Source: CAD feature listing. Evaluate the final solid. Frame: model axes, mm. Face numbers are marked on the shaded views. A direction names the side the tool comes from. Give positions to 0.01 mm unless a question says otherwise; leave off trailing zeros. Order: outer loops, then holes, each group sorted by start corner. A loop starts at its lowest first (then second) coordinate and runs counter-clockwise, first axis right, second up. Notation, with made-up numbers: M -0.75,23.25 L 41.25,23.25 A20 ccw 41.25,49.25 Z; hole C 32,-4 d9. An arc over 180 degrees is marked long. Use CSV: the item, a comma, the result in double quotes. Start each with the question number.
Item 1: Pull-direction query (X, two-part tool) for the marked faces 1, 2 and 3; classes: +X half, -X half, draft (parallel to the pull), parting line (faces both ways), or undercut.
Item 2: Section query A-A on y = 25.4. Return loops of the section in (x, z) (3 decimals).
Item 3: Section query C-C on x = 34. Return loops of the section in (y, z).
Item 4: First-contact query: pin 1 (8 mm diameter, centred on x = -3.5, y = 5, fed in from +Z); pin 2 (8 mm diameter, centred on x = -17, z = 72, fed in from +Y); pin 3 (1 mm diameter, centred on x = -32.5, y = 11, fed in from -Z); pin 4 (4 mm diameter, centred on x = 12.5, y = 14.5, fed in from +Z). Flat tips, straight axial feed; report the tip coordinate or a pass-through.
Item 5: Section query D-D on z = 47.5. Return loops of the section in (x, y).
Item 6: Section query B-B on x = 50.8. Return loops of the section in (y, z) (3 decimals), and give its area (3 significant figures).
Item 7: Access query for the marked faces 4 and 5. Directions: +Z, -Z, +X, -X, +Y, -Y. A direction counts if a zero-diameter tool reaches every point of the face in a straight line with its end or side. Return the directions, or none.
Item 8: Ray query, probe 1 along X at (y, z) = (25, 8); probe 2 along Y at (x, z) = (50.8, 8) (3 decimals); probe 3 along X at (y, z) = (-20.5, 4). Return the intervals inside material, ascending. Write a range as from..to.
from build123d import *

# Parameters (mm, degrees)
F0_W     = 127
F0_H     = 76.2
F1_DEPTH = 25.4
F3_D     = 19.05
F4_W     = 19.05
F4_H     = 50.8
F6_W     = 12.7
F6_H     = 25.4
F9_R     = 2.54


# Not quite as in the source:
# - a fillet or chamfer that OpenCascade refuses, or shapes differently, is made with other operations: its cross-section is extruded or revolved along the edge and cut away or added


with BuildPart() as f1:
    # F0 (on Top) → F1 (new body)
    with BuildSketch(Plane.XY):
        Rectangle(F0_W, F0_H)
    extrude(amount=F1_DEPTH)

    # F3 (through all)
    with Locations(Plane.XY.offset(25.4)):
        with Locations((-50.8, 25.4), (50.8, 25.4), (-50.8, -25.4), (50.8, -25.4)):
            Hole(F3_D / 2)

    # F4 (on Front) → F5 (revolve)
    with BuildSketch(Plane.XZ):
        with Locations((-9.525, 50.8)):
            Rectangle(F4_W, F4_H)
    revolve(axis=Axis((0, 0, 50.8), (0, 0, 1)))

    # F6 (on Front) → F7 (revolve, cut)
    with BuildSketch(Plane.XZ):
        with Locations((-19.05, 50.8)):
            Rectangle(F6_W, F6_H)
    revolve(axis=Axis((0, 0, 50.8), (0, 0, -1)), mode=Mode.SUBTRACT)

    # F8: fillet of radius 10.16 on 2 edges, made by hand

    # F8_s1 → F8_t2 (revolve, cut)
    with BuildSketch(Plane.XZ):
        with BuildLine():
            ThreePointArc((-19.05, 28.6814279214), (-17.3142269675, 34.3610405842), (-12.7, 38.1))
            Line((-12.7, 38.1), (-19.05, 38.1))
            Line((-19.05, 38.1), (-19.05, 28.6814279214))
        make_face()
    revolve(axis=Axis((0, 0, 38.1), (0, 0, -1)), mode=Mode.SUBTRACT)

    # F8_s3 → F8_t4 (revolve, cut)
    with BuildSketch(Plane.XZ):
        with BuildLine():
            ThreePointArc((-12.7, 63.5), (-17.3142269675, 67.2389594158), (-19.05, 72.9185720786))
            Line((-19.05, 72.9185720786), (-19.05, 63.5))
            Line((-19.05, 63.5), (-12.7, 63.5))
        make_face()
    revolve(axis=Axis((0, 0, 63.5), (0, 0, -1)), mode=Mode.SUBTRACT)

    # F9
    f9_edges = [f1.edges().sort_by_distance(p)[0] for p in [
        (0, 38.1, 25.4),
        (63.5, 0, 25.4),
        (0, -38.1, 25.4),
        (-63.5, 0, 25.4),
    ]]
    fillet(f9_edges, radius=F9_R)

    # F10: fillet of radius 5.08 on 1 edges, made by hand

    # F10_s1 → F10_t2 (revolve, cut)
    with BuildSketch(Plane.XZ):
        with BuildLine():
            ThreePointArc((-18.3919026469, 69.3214279214), (-17.8208524084, 74.0070100312), (-13.6409513235, 76.2))
            Line((-13.6409513235, 76.2), (-13.6409513235, 76.708))
            Line((-13.6409513235, 76.708), (-19.05, 76.708))
            Line((-19.05, 76.708), (-19.558, 76.2))
            ThreePointArc((-19.558, 76.2), (-19.558, 72.9185720786), (-18.8669977793, 69.1415707135))
            Line((-18.8669977793, 69.1415707135), (-18.3919026469, 69.3214279214))
        make_face()
    revolve(axis=Axis((0, 0, 76.2), (0, 0, 1)), mode=Mode.SUBTRACT)

    # F11 (on Front) → F12 (revolve)
    with BuildSketch(Plane.XZ):
        with BuildLine():
            Line((0, 76.2), (0, 89.8398))
            ThreePointArc((0, 89.8398), (-9.710461042, 85.7786789481), (-13.638526776, 76.0136363248))
            Line((-13.638526776, 76.0136363248), (0, 76.2))
        make_face()
    revolve(axis=Axis((0, 0, 83.0199), (0, 0, -1)))


solid = f1.part
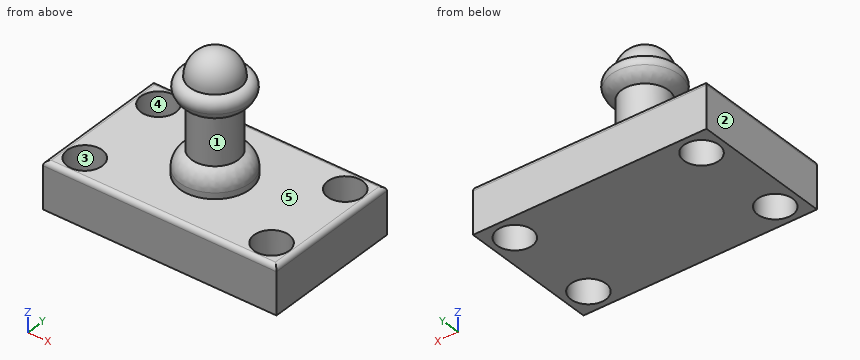
Verdict:
1,face 1,"parting line"
1,face 2,"-X half"
1,face 3,"undercut"
2,outline,"M -63.5,0 L -60.325,0 L -60.325,25.4 L -60.96,25.4 A2.54 ccw -63.5,22.86 Z; M -41.275,0 L 41.275,0 L 41.275,25.4 L -41.275,25.4 Z; M 60.325,0 L 63.5,0 L 63.5,22.86 A2.54 ccw 60.96,25.4 L 60.325,25.4 Z"
3,outline,"M -38.1,0 L 38.1,0 L 38.1,22.86 A2.54 ccw 35.56,25.4 L -35.56,25.4 A2.54 ccw -38.1,22.86 Z"
4,pin 1,"z = 89.68"
4,pin 2,"y = 13.42"
4,pin 3,"z = 0"
4,pin 4,"z = 74.8"
5,outline,"C 0,0 d25.4"
6,outline,"M -38.1,0 L -34.925,0 L -34.925,25.4 L -35.56,25.4 A2.54 ccw -38.1,22.86 Z; M -15.875,0 L 15.875,0 L 15.875,25.4 L -15.875,25.4 Z; M 34.925,0 L 38.1,0 L 38.1,22.86 A2.54 ccw 35.56,25.4 L 34.925,25.4 Z"
6,area,"965 mm2"
7,face 4,"+Z, -Z"
7,face 5,"+Z"
8,probe 1,"-63.5..-60.32, -41.28..41.28, 60.32..63.5"
8,probe 2,"-38.1..-34.925, -15.875..15.875, 34.925..38.1"
8,probe 3,"-63.5..-58.97, -42.63..42.63, 58.97..63.5"
